from build123d import *

# Parameters (mm, degrees)
ESBO_O2_W                = 13
ESBO_O2_H                = 9.6
RESSALTO_EXTRUS_O1_DEPTH = 7.7
ESBO_O3_R                = 2.8
RESSALTO_EXTRUS_O2_DEPTH = 8.8
ESBO_O5_R                = 1.4
RESSALTO_EXTRUS_O3_DEPTH = 10.5


with BuildPart() as part:
    # Esboço2 → Ressalto-extrusão1 (new body)
    with BuildSketch(Plane.XY):
        with Locations((6.5, 4.8)):
            Rectangle(ESBO_O2_W, ESBO_O2_H)
    extrude(amount=RESSALTO_EXTRUS_O1_DEPTH)

    # Esboço3 → Ressalto-extrusão2 (add)
    with BuildSketch(Plane(origin=(0, 9.6, 0), x_dir=(1, 0, 0), z_dir=(0, 1, 0))):
        with Locations(Location((6.5, -3.85, 0), (0, 0, 270))):
            Circle(ESBO_O3_R)
    extrude(amount=RESSALTO_EXTRUS_O2_DEPTH)

    # Esboço5 → Ressalto-extrusão3 (add)
    with BuildSketch(Plane(origin=(0, 18.4, 0), x_dir=(1, 0, 0), z_dir=(0, 1, 0))):
        with Locations(Location((6.5, -3.85, 0), (0, 0, 90))):
            Circle(ESBO_O5_R)
    extrude(amount=RESSALTO_EXTRUS_O3_DEPTH)


solid = part.part
Part model, mm, in its own coordinate system. A direction names the side the tool comes from. Round coordinates to 2 decimals unless told otherwise and drop trailing zeros. Loops run counter-clockwise (first coordinate to the right, second up) from the corner with the lowest first, then second, coordinate; pieces in that order, holes last. Notation, with made-up numbers: (49, 72) - (108, 72) arc R28 ccw to (108, 91) - close; hole circle Ø11 at (70.5, 28.25). An arc over 180 degrees is marked (long way). Answer as a JSON object with one key per item and string values.
Item 1: Band-saw the part on A-A on z = 3.85. List the corners of the cut face in (x, y).
Output:
{"outline": "(0, 0) - (13, 0) - (13, 9.6) - (9.3, 9.6) - (9.3, 18.4) - (7.9, 18.4) - (7.9, 28.9) - (5.1, 28.9) - (5.1, 18.4) - (3.7, 18.4) - (3.7, 9.6) - (0, 9.6) - close"}
Item 2: Tool access for faces 1 (the face through (7.04, 23.58, 2.56)), 2 (the face through (6, 5, 0)): list every direction of +Z, -Z, +X, -X, +Y, -Y with a clear straight run to the whole face (end or side of a thin tool).
Output:
{"face 1": "+Y", "face 2": "-Z, +X, -X, +Y, -Y"}
Item 3: Wall check: L1, parallel to Y at x = 2, z = 3; L2, parallel to Y at x = 6.75, z = 2.25; L3, parallel to X at y = 15.75, z = 4. Give the ranges that are in metal, low to high.
Output:
{"L1": "0 to 9.6", "L2": "0 to 18.4", "L3": "3.7 to 9.3"}
Item 4: Band-saw the part on C-C on y = 15.5. List the corners of the cut face in (x, z), plus the area to 3 significant figures.
Output:
{"outline": "circle Ø5.6 at (6.5, 3.85)", "area": "24.6 mm2"}
Item 5: Band-saw the part on B-B on x = 6.5. List the corners of the cut face in (y, z).
Output:
{"outline": "(0, 0) - (9.6, 0) - (9.6, 1.05) - (18.4, 1.05) - (18.4, 2.45) - (28.9, 2.45) - (28.9, 5.25) - (18.4, 5.25) - (18.4, 6.65) - (9.6, 6.65) - (9.6, 7.7) - (0, 7.7) - close"}
Item 6: Pin check, flat tips, straight feed: pin 1 (1 mm diameter, centred on x = 8.5, y = 14.5, fed in from -Z); pin 2 (1.5 mm diameter, centred on y = 15.5, z = 5, fed in from -X); pin 3 (4 mm diameter, centred on x = 3, z = 5, fed in from +Y). Stop position of each tip, or through.
Output:
{"pin 1": "z = 1.49", "pin 2": "x = 3.73", "pin 3": "y = 18.4"}
Item 7: Band-saw the part on D-D on z = 6.25. List the corners of the cut face in (x, y).
Output:
{"outline": "(0, 0) - (13, 0) - (13, 9.6) - (7.94, 9.6) - (7.94, 18.4) - (5.06, 18.4) - (5.06, 9.6) - (0, 9.6) - close"}
